The listing builds one solid part. Answer for the finished solid, in the listing's coordinates (mm). A direction names the side the tool comes from. Round coordinates to 2 decimals unless told otherwise and drop trailing zeros. Write each loop counter-clockwise with the first axis right and the second up, starting at its lowest first coordinate (ties: lowest second). Pieces come first, ordered by that corner, then holes. Notation, with made-up numbers: (-32, 19) - (23, 19) arc R17 ccw to (23, 41) - close; hole circle Ø9 at (21, 64.5). An arc over 180 degrees is marked (long way). Answer as CSV lines item,"result". Start each with the question number.
Item 1: Which of the six approach directions +Z, -Z, +X, -X, +Y, -Y give full straight-line access (tool end or side, diameter ignored) to faces 1 (the flat face through (-2, 12, 0)), 2 (the flat face through (-18, 3, 17)), 3 (the flat face through (-2, 23, 5.5))?
Item 2: A cutting plane is placed at C-C on z = 27. Determine the outline of the cut face in (x, y), and give its area (3 significant figures).
Item 3: A cutting plane is placed at B-B on y = 11.5. Determine the outline of the cut face in (x, z).
Item 4: A cutting plane is placed at A-A on y = 19. Determine the outline of the cut face in (x, z).
Item 5: Straight lines are drawn through the part: line 1 along Y through (x, z) = (-2, 31.5); line 2 along Y through (x, z) = (-1.5, 15); line 3 along Y through (x, z) = (-1, 3). For each, find the intervals that lie inside material, in ascending order. Write a range as [from, to].
Item 6: For a pull along Z with two mould halves and no side action, classify faces 4 (the flat face through (-2, 12, 35)), 5 (the flat face through (-1, 43, 17)), 6 (the cylindrical face through (-1.521, 14.024, 3.283)) as pulls with the +Z half, pulls with the -Z half, needs draft (parallel to the pull), parting line crosses it, or undercut.
Item 7: A cutting plane is placed at D-D on x = -24.5. Determine the outline of the cut face in (y, z), and give its area (3 significant figures).
Item 8: Flat-ended cylindrical pins translate along their axes: pin 1 (1.5 mm diameter, centred on x = -11.5, z = 14, fed in from -Y); pin 2 (2.5 mm diameter, centred on y = 31, z = 31.5, fed in from -X); pin 3 (1 mm diameter, centred on x = -18, z = 7.5, fed in from +Y). Find the tip coordinate at first contact, or state that the pin passes through.
```python
from build123d import *

# Parameters (mm, degrees)
EXTRUDE_1_DEPTH     = 35
SKETCH_2_W          = 24
SKETCH_2_H          = 32
SKETCH_2_R          = 1
CUT_EXTRUDE_1_DEPTH = 4
SKETCH_3_R          = 1.5
CUT_EXTRUDE_2_DEPTH = 4


with BuildPart() as part:
    # 草图1 → 凸台-拉伸1 (new body)
    with BuildSketch(Plane.XY):
        Polygon((-33, 0), (0, 0), (0, 43), (-3, 43), (-3, 3), (-33, 3), align=None)
    extrude(amount=EXTRUDE_1_DEPTH)

    # 草图2 → 切除-拉伸1 (cut, through all)
    with BuildSketch(Plane.ZY.offset(3)):
        with Locations((17.5, 23)):
            Rectangle(SKETCH_2_W, SKETCH_2_H)
        with Locations((3.5, 31)):
            Circle(SKETCH_2_R)
        with Locations((3.5, 27)):
            Circle(SKETCH_2_R)
        with Locations((3.5, 23)):
            Circle(SKETCH_2_R)
        with Locations((3.5, 19)):
            Circle(SKETCH_2_R)
        with Locations((3.5, 15)):
            Circle(SKETCH_2_R)
        with Locations((31.5, 15)):
            Circle(SKETCH_2_R)
        with Locations((31.5, 19)):
            Circle(SKETCH_2_R)
        with Locations((31.5, 23)):
            Circle(SKETCH_2_R)
        with Locations((31.5, 27)):
            Circle(SKETCH_2_R)
        with Locations((31.5, 31)):
            Circle(SKETCH_2_R)
    extrude(amount=-CUT_EXTRUDE_1_DEPTH, mode=Mode.SUBTRACT)

    # 草图3 → 切除-拉伸2 (cut, through all)
    with BuildSketch(Plane(origin=(0, 3, 0), x_dir=(1, 0, 0), z_dir=(0, 1, 0))):
        with Locations((-25.310950673, -8)):
            Circle(SKETCH_3_R)
        with Locations((-10.689049327, -8)):
            Circle(SKETCH_3_R)
        with Locations((-10.689049327, -27)):
            Circle(SKETCH_3_R)
        with Locations((-25.310950673, -27)):
            Circle(SKETCH_3_R)
    extrude(amount=-CUT_EXTRUDE_2_DEPTH, mode=Mode.SUBTRACT)


solid = part.part
```
Geometry says:
1,face 1,"-Z, +X, -X, +Y, -Y"
1,face 2,"+Z, -Z, -X, +Y"
1,face 3,"+X, -X"
2,outline,"(-33, 0) - (-26.81, 0) - (-26.81, 3) - (-33, 3) - close; (-23.81, 0) - (-12.19, 0) - (-12.19, 3) - (-23.81, 3) - close; (-9.19, 0) - (0, 0) - (0, 7) - (-3, 7) - (-3, 3) - (-9.19, 3) - close; (-3, 39) - (0, 39) - (0, 43) - (-3, 43) - close"
2,area,"105 mm^2"
3,outline,"(-3, 0) - (0, 0) - (0, 5.5) - (-3, 5.5) - close; (-3, 29.5) - (0, 29.5) - (0, 35) - (-3, 35) - close"
4,outline,"(-3, 0) - (0, 0) - (0, 2.5) - (-3, 2.5) - close; (-3, 4.5) - (0, 4.5) - (0, 5.5) - (-3, 5.5) - close; (-3, 29.5) - (0, 29.5) - (0, 30.5) - (-3, 30.5) - close; (-3, 32.5) - (0, 32.5) - (0, 35) - (-3, 35) - close"
5,line 1,"y = [0, 14], [16, 18], [20, 22], [24, 26], [28, 30], [32, 43]"
5,line 2,"y = [0, 7], [39, 43]"
5,line 3,"y = [0, 14.13], [15.87, 18.13], [19.87, 22.13], [23.87, 26.13], [27.87, 30.13], [31.87, 43]"
6,face 4,"pulls with the +Z half"
6,face 5,"needs draft"
6,face 6,"undercut"
7,outline,"(0, 0) - (3, 0) - (3, 6.74) - (0, 6.74) - close; (0, 9.26) - (3, 9.26) - (3, 25.74) - (0, 25.74) - close; (0, 28.26) - (3, 28.26) - (3, 35) - (0, 35) - close"
7,area,"89.9 mm^2"
8,pin 1,"stops at y = 0"
8,pin 2,"stops at x = -3"
8,pin 3,"stops at y = 3"
